Input: part model. Units: mm. Frame: model coordinates. Face numbers are marked on the shaded views. A direction names the side the tool comes from. Round coordinates to 2 decimals unless told otherwise and drop trailing zeros. Loops run counter-clockwise (first coordinate to the right, second up) from the corner with the lowest first, then second, coordinate; pieces in that order, holes last.
1) First-contact query: pin 1 (1.5 mm diameter, centred on y = -8.5, z = 1, fed in from +X); pin 2 (1.5 mm diameter, centred on x = 1.5, z = 2, fed in from +Y); pin 3 (1.5 mm diameter, centred on x = -0.5, y = -3, fed in from -Z); pin 4 (1.5 mm diameter, centred on y = -7.5, z = 2.5, fed in from -X). Flat tips, straight axial feed; report the tip coordinate or a pass-through.
2) Section C-C, the plane x = 2.25. Return loops of the section in (y, z).
3) Ray query, line 1 along X through (y, z) = (-10.5, 4.15); line 2 along X through (y, z) = (0, 3.5) (3 decimals); line 3 along Y through (x, z) = (-3.5, 0.35). Return the intervals inside material, ascending.
4) Section D-D, the plane x = 0. Return loops of the section in (y, z) (3 decimals).
5) Access query for the marked faces 1, 2 and 3. Directions: +Z, -Z, +X, -X, +Y, -Y. A direction counts if a zero-diameter tool reaches every point of the face in a straight line with its end or side. Return the directions, or none.
6) Section A-A, the plane y = -13. Return loops of the section in (x, z).
7) Section B-B, the plane z = 1.35. Return loops of the section in (x, y) (3 decimals), and give its area (3 significant figures).
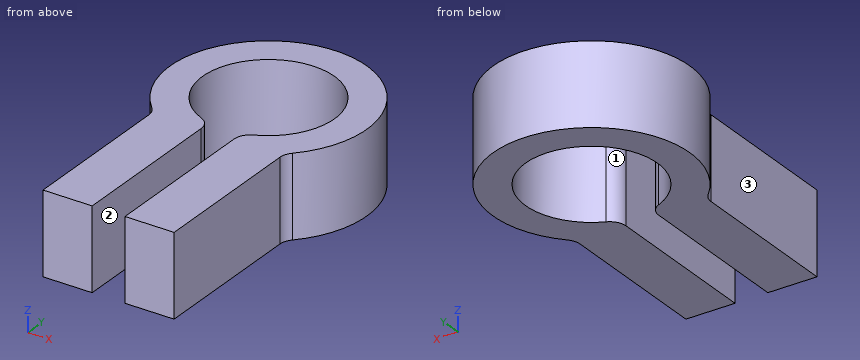
from build123d import *

# Parameters (mm, degrees)
BOSS_EXTRUDE1_DEPTH = 5
FILLET1_R           = 1


with BuildPart() as part:
    # Sketch1 → Boss-Extrude1 (new body)
    with BuildSketch(Plane.XY):
        with BuildLine():
            Line((-1, -3.898797892), (-1, -14.472135955))
            Line((-1, -14.472135955), (-4, -14.472135955))
            Line((-4, -14.472135955), (-4, -4.472135955))
            ThreePointArc((-4, -4.472135955), (0, 6), (4, -4.472135955))
            Line((4, -4.472135955), (4, -14.472135955))
            Line((4, -14.472135955), (1, -14.472135955))
            Line((1, -14.472135955), (1, -3.898797892))
            ThreePointArc((1, -3.898797892), (0, 4.025), (-1, -3.898797892))
        make_face()
    extrude(amount=BOSS_EXTRUDE1_DEPTH)

    # Fillet1
    fillet1_edges = [part.edges().sort_by_distance(p)[0] for p in [
        (-1, -3.898797892, 2.5),
        (-4, -4.472135955, 2.5),
        (4, -4.472135955, 2.5),
        (1, -3.898797892, 2.5),
    ]]
    fillet(fillet1_edges, radius=FILLET1_R)


solid = part.part
Final values:
1. pin 1: stops at x = 4
1. pin 2: stops at y = 5.95
1. pin 3: passes through
1. pin 4: stops at x = -4
2. outline: (-14.47, 0) - (-3.34, 0) - (-3.34, 5) - (-14.47, 5) - close; (3.34, 0) - (5.56, 0) - (5.56, 5) - (3.34, 5) - close
3. line 1: x = -4 to -1, 1 to 4
3. line 2: x = -6 to -4.025, 4.025 to 6
3. line 3: y = -14.47 to -1.99, 1.99 to 4.87
4. outline: (4.025, 0) - (6, 0) - (6, 5) - (4.025, 5) - close
5. face 1: +Z, -Z
5. face 2: +Z, -Z, -Y
5. face 3: +Z, -Z, -X, -Y
6. outline: (-4, 0) - (-1, 0) - (-1, 5) - (-4, 5) - close; (1, 0) - (4, 0) - (4, 5) - (1, 5) - close
7. outline: (-4.286, -4.199) arc R1 cw to (-4, -4.899) - (-4, -14.472) - (-1, -14.472) - (-1, -4.61) arc R1 ccw to (-1.602, -3.692) arc R4.025 cw (long way) to (1.602, -3.692) arc R1 ccw to (1, -4.61) - (1, -14.472) - (4, -14.472) - (4, -4.899) arc R1 cw to (4.286, -4.199) arc R6 ccw (long way) to start
7. area: 113 mm2
